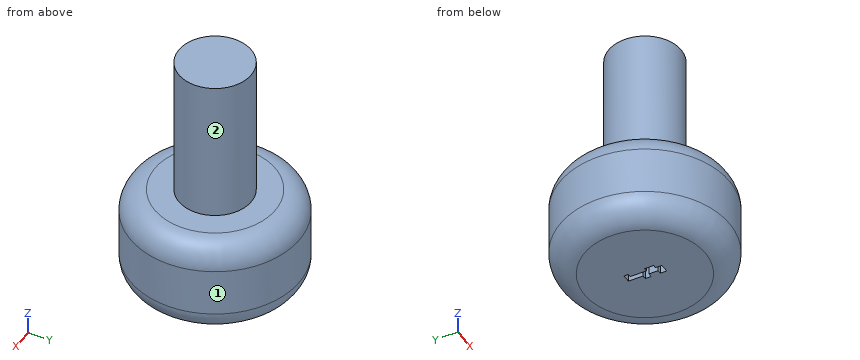
from build123d import *

# Parameters (mm, degrees)
F0_R     = 88.9
F0_R_2   = 38.1
F1_DEPTH = 101.6
F2_DEPTH = 254
F3_R     = 25.4
F4_R     = 25.4
F6_DEPTH = 50.8


with BuildPart() as f1:
    # F0 (on Top) → F1 (new body)
    with BuildSketch(Plane.XY):
        Circle(F0_R)
        Circle(F0_R_2, mode=Mode.SUBTRACT)
    extrude(amount=F1_DEPTH)

    # F0 (on Top) → F2 (join)
    with BuildSketch(Plane.XY):
        Circle(F0_R_2)
    extrude(amount=F2_DEPTH)

    # F3
    f3_edges = [f1.edges().sort_by_distance(p)[0] for p in [
        (-88.9, 0, 101.6),
    ]]
    fillet(f3_edges, radius=F3_R)

    # F4
    f4_edges = [f1.edges().sort_by_distance(p)[0] for p in [
        (-88.9, 0, 0),
    ]]
    fillet(f4_edges, radius=F4_R)

    # F5 (on face) → F6 (cut)
    with BuildSketch(Plane(origin=(0, 0, 0), x_dir=(1, 0, 0), z_dir=(0, 0, -1))):
        Polygon((6.030925, 19.711075), (-3.144438, 19.711075), (-3.144438, 12.908415), (-6.669075, 12.908415), (-6.669075, 3.30908), (-3.144438, 3.30908), (-3.144438, -13.90423), (-6.669075, -13.90423), (-6.669075, -18.388925), (1.821126, -18.388925), (1.821126, -2.981285), (6.030925, -2.981285), (6.030925, 3.30908), (1.821126, 3.30908), (1.821126, 12.908415), (6.030925, 12.908415), align=None)
    extrude(amount=-F6_DEPTH, mode=Mode.SUBTRACT)


solid = f1.part
Could you check a few things on this model? Use its own coordinates, in mm. Face numbers are marked on the shaded views. A direction names the side the tool comes from. Give positions to 0.01 mm unless a question says otherwise; leave off trailing zeros. Write each loop counter-clockwise with the first axis right and the second up, starting at its lowest first coordinate (ties: lowest second). Pieces come first, ordered by that corner, then holes. Notation, with made-up numbers: (20.25, -16.5) -> (75.25, -16.5) arc R15 cw to (75.25, 8.5) -> close; hole circle Ø5 at (37, 11.5). An arc over 180 degrees is marked (long way). Answer as CSV lines item,"result". Start each with the question number.
(1) Please list where these lines run through material, in increasing order: line 1 (Z direction, x = 33.5, y = 49); line 2 (Z direction, x = 1.5, y = -9); line 3 (X direction, y = 2.5, z = 22).
(2) If we section it at A-A, the plane z = 20.5: Write out the boundary of the cut face in (x, y), and give its area (3 significant figures).
(3) If we section it at C-C, the plane z = 209.5: Write out the boundary of the cut face in (x, y), and give its area (3 significant figures).
(4) Which directions (+Z, -Z, +X, -X, +Y, -Y) give clear straight access to the entire face, cutting with the end or side of a thin tool? Please do the marked faces 1 and 2.
(5) I'm going to push flat-ended pins straight in: pin 1 Ø1.8 at (x, z) = (-5.5, 34.5) entering from -Y; pin 2 Ø2.5 at (x, z) = (-1, 21) entering from -Y; pin 3 Ø3.5 at (x, z) = (3, 23.5) entering from -Y. Where does each tip first touch, or does it pass through?
(6) If we section it at B-B, the plane y = 0: Write out the boundary of the cut face in (x, z), and give its area (3 significant figures).
Answer list:
1,line 1,"0 to 101.6"
1,line 2,"50.8 to 254"
1,line 3,"-88.64 to -3.14, 6.03 to 88.64"
2,outline,"circle Ø176.85 at (0, 0); hole (-6.67, -12.91) -> (-3.14, -12.91) -> (-3.14, -19.71) -> (6.03, -19.71) -> (6.03, -12.91) -> (1.82, -12.91) -> (1.82, -3.31) -> (6.03, -3.31) -> (6.03, 2.98) -> (1.82, 2.98) -> (1.82, 18.39) -> (-6.67, 18.39) -> (-6.67, 13.9) -> (-3.14, 13.9) -> (-3.14, -3.31) -> (-6.67, -3.31) -> close"
2,area,"24,300 mm^2"
3,outline,"circle Ø76.2 at (0, 0)"
3,area,"4,560 mm^2"
4,face 1,"+Z, -Z"
4,face 2,"+Z"
5,pin 1,"y = -88.78"
5,pin 2,"y = -88.7"
5,pin 3,"y = -88.87"
6,outline,"(-88.9, 25.4) arc R25.4 ccw to (-63.5, 0) -> (-3.14, 0) -> (-3.14, 50.8) -> (6.03, 50.8) -> (6.03, 0) -> (63.5, 0) arc R25.4 ccw to (88.9, 25.4) -> (88.9, 76.2) arc R25.4 ccw to (63.5, 101.6) -> (38.1, 101.6) -> (38.1, 254) -> (-38.1, 254) -> (-38.1, 101.6) -> (-63.5, 101.6) arc R25.4 ccw to (-88.9, 76.2) -> close"
6,area,"28,700 mm^2"
